Source: CAD feature listing. Evaluate the final solid. Frame: model axes, mm. A direction names the side the tool comes from. Round coordinates to 2 decimals unless told otherwise and drop trailing zeros. Write each loop counter-clockwise with the first axis right and the second up, starting at its lowest first coordinate (ties: lowest second). Pieces come first, ordered by that corner, then holes.
Autodesk Inventor part; units mm, degrees
ref_plane "YZ Plane" through (0, 0, 0) normal (1, 0, 0) x (0, 1, 0)
ref_plane "XZ Plane" through (0, 0, 0) normal (0, 1, 0) x (-1, 0, 0)
ref_plane "XY Plane" through (0, 0, 0) normal (0, 0, 1) x (1, 0, 0)
ref_plane "Work Plane1" through (0, 0.2202, 0) normal (0, 0, 1) x (1, 0, 0)
sketch "Sketch1" plane through (0, 0.2202, 0) normal (0, 0, 1) x (1, 0, 0)
  line L0 (21.9247, 42.5927) -> (36.4247, 42.5927)
  line L1 (36.4247, 42.5927) -> (36.4247, 36.8927)
  line L2 (36.4247, 36.8927) -> (21.9247, 36.8927)
  line L3 (21.9247, 36.8927) -> (21.9247, 42.5927)
  point P0 (0, -0.2202)
  dimension "d0" = 14.5
  dimension "d2" = 5.7
extrude "Extrusion1" add sketch "Sketch1" along normal blind 13.2
sketch "Sketch2" plane through (36.4247, 37.1129, 0) normal (1, 0, 0) x (0, 0, -1)
  line L0 (0, 5.7) -> (0, 0)
  line L1 (0, 5.7) -> (-13.2, 5.7)
  line L2 (-13.2, 0) -> (-13.2, 5.7)
  line L3 (0, 0) -> (-13.2, 0)
  line L4 (-12.8, 5.3) -> (-0.4, 5.3)
  line L5 (-0.4, 5.3) -> (-0.4, 0.4)
  line L6 (-0.4, 0.4) -> (-12.8, 0.4)
  line L7 (-12.8, 0.4) -> (-12.8, 5.3)
  point P0 (0, -37.1129)
  dimension "d5" = 0.4
extrude "Extrusion2" cut sketch "Sketch2" against normal blind 13 contours L4 L5 L6 L7
sketch "Sketch3" plane through (23.4247, 37.1129, 0) normal (1, 0, 0) x (0, 0, -1)
  line L0 (-12.8, 0.4) -> (-12.8, 5.3)
  line L1 (-0.4, 0.4) -> (-12.8, 0.4)
  line L2 (-0.4, 5.3) -> (-0.4, 0.4)
  line L3 (-12.6, 2) -> (-0.6, 2)
  line L4 (-0.6, 2) -> (-0.6, 0.6)
  line L5 (-0.6, 0.6) -> (-12.6, 0.6)
  line L6 (-12.6, 0.6) -> (-12.6, 2)
  point P0 (0, -37.1129)
  dimension "d8" = 0.2
  dimension "d9" = 0.2
  dimension "d10" = 0.2
  dimension "d11" = 1.4
extrude "Extrusion3" add sketch "Sketch3" along normal blind 13
properties part number "nanopc_t4_usb"
1) Material intervals for line 1 (Y direction, x = 31, z = 9.5); line 2 (Z direction, x = 31, y = 38.6); line 3 (Z direction, x = 27, y = 37.55), sorted ascending.
Taken from the geometry:
line 1: y = 37.11 to 37.51, 37.71 to 39.11, 42.41 to 42.81
line 2: z = 0 to 0.4, 0.6 to 12.6, 12.8 to 13.2
line 3: z = 0 to 0.4, 12.8 to 13.2
2) Section query C-C on z = 8. Return the cut outline in (x, y), then the cut area to 4 significant figures.
Taken from the geometry:
outline: (21.92, 37.11) - (36.42, 37.11) - (36.42, 37.51) - (23.42, 37.51) - (23.42, 37.71) - (36.42, 37.71) - (36.42, 39.11) - (23.42, 39.11) - (23.42, 42.41) - (36.42, 42.41) - (36.42, 42.81) - (21.92, 42.81) - close
area: 37.15 mm2
3) Reachability of faces 1 (the face through (29, 40, 0)), 2 (the face through (30, 38, 0.6)) from +Z, -Z, +X, -X, +Y, -Y: full face, straight path, thin tool, end or side. Return the list, or none.
Taken from the geometry:
face 1: -Z, +X, -X, +Y, -Y
face 2: +X
4) Section query B-B on y = 40.35. Return the cut outline in (x, z), then the cut area to 3 significant figures.
Taken from the geometry:
outline: (21.92, 0) - (36.42, 0) - (36.42, 0.4) - (23.42, 0.4) - (23.42, 12.8) - (36.42, 12.8) - (36.42, 13.2) - (21.92, 13.2) - close
area: 30.2 mm2
5) Section query D-D on y = 38.35. Return the cut outline in (x, z).
Taken from the geometry:
outline: (21.92, 0) - (36.42, 0) - (36.42, 0.4) - (23.42, 0.4) - (23.42, 0.6) - (36.42, 0.6) - (36.42, 12.6) - (23.42, 12.6) - (23.42, 12.8) - (36.42, 12.8) - (36.42, 13.2) - (21.92, 13.2) - close
6) Section query A-A on x = 30.75. Return the cut outline in (y, z).
Taken from the geometry:
outline: (37.11, 0) - (42.81, 0) - (42.81, 13.2) - (37.11, 13.2) - close; (37.71, 0.6) - (39.11, 0.6) - (39.11, 12.6) - (37.71, 12.6) - close; hole (37.51, 0.4) - (42.41, 0.4) - (42.41, 12.8) - (37.51, 12.8) - close
7) Pull-direction query (Y, two-part tool) for faces 3 (the face through (29, 37.113, 7)), 4 (the face through (30, 37.713, 7)), 5 (the face through (36.425, 38, 7)); classes: released by +Y, released by -Y, zero draft, split by the parting line, or undercut.
Taken from the geometry:
face 3: released by -Y
face 4: undercut
face 5: zero draft
8) Contact query for flat-ended pins moving along their axis: P1, Ø3, axis at y = 40, z = 4.5, coming from the +X side; P2, Ø1.5, axis at y = 40.5, z = 4.5, coming from the +X side. Output: stop coordinate, or through.
Taken from the geometry:
P1: stops at x = 36.42
P2: stops at x = 23.42
